from build123d import *

# Parameters (mm, degrees)
MAIN_SKETCH_W                                  = 78
MAIN_SKETCH_H                                  = 16
MAIN_SKETCH_W_2                                = 72
MAIN_SKETCH_H_2                                = 9.5
MAIN_EXTRUSION_DEPTH                           = 100
FRAISAGE_POUR_VIS_T_TE_FRAIS_E_M31_D           = 3.4
FRAISAGE_POUR_VIS_T_TE_FRAIS_E_M31_CSINK_D     = 6.3
FRAISAGE_POUR_VIS_T_TE_FRAIS_E_M31_CSINK_ANGLE = 90
R_P_TITION_LIN_AIRE1_COUNT                     = 2
R_P_TITION_LIN_AIRE1_PITCH                     = 76.6
FRAISAGE_POUR_VIS_T_TE_FRAIS_E_M32_D           = 3.4
FRAISAGE_POUR_VIS_T_TE_FRAIS_E_M32_CSINK_D     = 6.3
FRAISAGE_POUR_VIS_T_TE_FRAIS_E_M32_CSINK_ANGLE = 90
R_P_TITION_LIN_AIRE3_COUNT                     = 2
R_P_TITION_LIN_AIRE3_PITCH                     = 76.5
FRAISAGE_POUR_VIS_T_TE_FRAIS_E_M33_D           = 3.4
FRAISAGE_POUR_VIS_T_TE_FRAIS_E_M33_CSINK_D     = 6.3
FRAISAGE_POUR_VIS_T_TE_FRAIS_E_M33_CSINK_ANGLE = 90
SUPPORT_FIX_HOLE_REACH                         = 18
SUPPORT_FIX_SKETCH_R                           = 1.35


with BuildPart() as part:
    # Main-Sketch → Main-Extrusion (new body)
    with BuildSketch(Plane.XY):
        with Locations((39, 8)):
            Rectangle(MAIN_SKETCH_W, MAIN_SKETCH_H)
        with Locations((39, 8)):
            Rectangle(MAIN_SKETCH_W_2, MAIN_SKETCH_H_2, mode=Mode.SUBTRACT)
    extrude(amount=MAIN_EXTRUSION_DEPTH)

    # Fraisage pour vis à tête fraisée M31 (through all)
    with Locations(Plane.ZY):
        with Locations((9, 9.5)):
            fraisage_pour_vis_t_te_frais_e_m31 = CounterSinkHole(FRAISAGE_POUR_VIS_T_TE_FRAIS_E_M31_D / 2, FRAISAGE_POUR_VIS_T_TE_FRAIS_E_M31_CSINK_D / 2, counter_sink_angle=FRAISAGE_POUR_VIS_T_TE_FRAIS_E_M31_CSINK_ANGLE)

    # Répétition linéaire1: Fraisage pour vis à tête fraisée M31 ×2
    with Locations(*[(0, 0, i * R_P_TITION_LIN_AIRE1_PITCH) for i in range(1, R_P_TITION_LIN_AIRE1_COUNT)]):
        add(fraisage_pour_vis_t_te_frais_e_m31, mode=Mode.SUBTRACT)

    # Fraisage pour vis à tête fraisée M32 (through all)
    with Locations(Plane(origin=(78, 0, 0), x_dir=(0, 0, -1), z_dir=(1, 0, 0))):
        with Locations((-85.6, 9.5)):
            fraisage_pour_vis_t_te_frais_e_m32 = CounterSinkHole(FRAISAGE_POUR_VIS_T_TE_FRAIS_E_M32_D / 2, FRAISAGE_POUR_VIS_T_TE_FRAIS_E_M32_CSINK_D / 2, counter_sink_angle=FRAISAGE_POUR_VIS_T_TE_FRAIS_E_M32_CSINK_ANGLE)

    # Répétition linéaire3: Fraisage pour vis à tête fraisée M32 ×2
    with Locations(*[(i * R_P_TITION_LIN_AIRE3_PITCH, 0, 0) for i in range(1, R_P_TITION_LIN_AIRE3_COUNT)]):
        add(fraisage_pour_vis_t_te_frais_e_m32, mode=Mode.SUBTRACT)

    # Fraisage pour vis à tête fraisée M33 (through all)
    with Locations(Plane(origin=(78, 0, 0), x_dir=(0, 0, -1), z_dir=(1, 0, 0))):
        with Locations((-9, 9.5)):
            CounterSinkHole(FRAISAGE_POUR_VIS_T_TE_FRAIS_E_M33_D / 2, FRAISAGE_POUR_VIS_T_TE_FRAIS_E_M33_CSINK_D / 2, counter_sink_angle=FRAISAGE_POUR_VIS_T_TE_FRAIS_E_M33_CSINK_ANGLE)

    # Support-Fix-Sketch → Support-Fix-Hole (cut, up to next)
    with BuildSketch(Plane.XZ, mode=Mode.PRIVATE) as support_fix_hole_sk1:
        with Locations((68, 90)):
            Circle(SUPPORT_FIX_SKETCH_R)
    support_fix_hole_tool1 = extrude(support_fix_hole_sk1.sketch, amount=-SUPPORT_FIX_HOLE_REACH, mode=Mode.PRIVATE) & part.part
    add(support_fix_hole_tool1.solids().sort_by_distance((68, 0, 90))[0], mode=Mode.SUBTRACT)
    # Support-Fix-Sketch → Support-Fix-Hole (cut, up to next)
    with BuildSketch(Plane.XZ, mode=Mode.PRIVATE) as support_fix_hole_sk2:
        with Locations((68, 10)):
            Circle(SUPPORT_FIX_SKETCH_R)
    support_fix_hole_tool2 = extrude(support_fix_hole_sk2.sketch, amount=-SUPPORT_FIX_HOLE_REACH, mode=Mode.PRIVATE) & part.part
    add(support_fix_hole_tool2.solids().sort_by_distance((68, 0, 10))[0], mode=Mode.SUBTRACT)
    # Support-Fix-Sketch → Support-Fix-Hole (cut, up to next)
    with BuildSketch(Plane.XZ, mode=Mode.PRIVATE) as support_fix_hole_sk3:
        with Locations((10, 10)):
            Circle(SUPPORT_FIX_SKETCH_R)
    support_fix_hole_tool3 = extrude(support_fix_hole_sk3.sketch, amount=-SUPPORT_FIX_HOLE_REACH, mode=Mode.PRIVATE) & part.part
    add(support_fix_hole_tool3.solids().sort_by_distance((10, 0, 10))[0], mode=Mode.SUBTRACT)
    # Support-Fix-Sketch → Support-Fix-Hole (cut, up to next)
    with BuildSketch(Plane.XZ, mode=Mode.PRIVATE) as support_fix_hole_sk4:
        with Locations((10, 90)):
            Circle(SUPPORT_FIX_SKETCH_R)
    support_fix_hole_tool4 = extrude(support_fix_hole_sk4.sketch, amount=-SUPPORT_FIX_HOLE_REACH, mode=Mode.PRIVATE) & part.part
    add(support_fix_hole_tool4.solids().sort_by_distance((10, 0, 90))[0], mode=Mode.SUBTRACT)


solid = part.part
Could you check a few things on this model? Use its own coordinates, in mm. A direction names the side the tool comes from. Coordinates: 2 decimals unless noted, no trailing zeros. Write each loop counter-clockwise with the first axis right and the second up, starting at its lowest first coordinate (ties: lowest second). Pieces come first, ordered by that corner, then holes. Notation, with made-up numbers: (15.5, -15.75) - (26.5, -15.75) arc R18 ccw to (26.5, 1.25) - close; hole circle Ø10 at (-30.5, 46.5). An arc over 180 degrees is marked (long way). Write item = value, one per line.
1) Suppose I cut it at A-A on x = 68. Please give me the cut outline in (y, z), plus the area to 3 significant figures.
Result set:
outline = (0, 0) - (3.25, 0) - (3.25, 8.65) - (0, 8.65) - close; (0, 11.35) - (3.25, 11.35) - (3.25, 88.65) - (0, 88.65) - close; (0, 91.35) - (3.25, 91.35) - (3.25, 100) - (0, 100) - close; (12.75, 0) - (16, 0) - (16, 100) - (12.75, 100) - close
area = 632 mm2
2) Please list where these lines run through material, in increasing order: line 1 (Z direction, x = 2.3, y = 9.5); line 2 (Z direction, x = 68, y = 1.2); line 3 (X direction, y = 1.8, z = 90). Write a range as [from, to].
Result set:
line_1 = [0, 7.3], [10.7, 83.9], [87.3, 100]
line_2 = [0, 8.65], [11.35, 88.65], [91.35, 100]
line_3 = [0, 8.65], [11.35, 66.65], [69.35, 78]
3) Suppose I cut it at C-C on y = 9.5. State how many separate pieces and enclosed holes the cut face has, plus the area to 3 significant figures.
Result set:
separate_pieces = 6
enclosed_holes = 0
area = 551 mm2
4) Suppose I cut it at D-D on x = 55. Please give me the cut outline in (y, z).
Result set:
outline = (0, 0) - (3.25, 0) - (3.25, 100) - (0, 100) - close; (12.75, 0) - (16, 0) - (16, 100) - (12.75, 100) - close
5) We'd pull the mould along X, two halves only. Please class faces 1 (the flat face through (38, 3.25, 49)), 2 (the flat face through (3, 8, 49)), 3 (the flat face through (38, 16, 49)), 4 (the flat face through (0, 8, 49)): +X half, -X half, draft (parallel to the pull), parting line (faces both ways), or undercut.
Result set:
face_1 = undercut
face_2 = undercut
face_3 = draft
face_4 = -X half
6) For faces 5 (the flat face through (38, 3, 0)), 6 (the cylindrical face through (10.62, 1.6, 88.8)), which set-ups out of +Z, -Z, +X, -X, +Y, -Y let a thin tool reach every point of the face, with its end or its side?
Result set:
face_5 = -Z, +X, -X, +Y, -Y
face_6 = -Y
7) Suppose I cut it at B-B on z = 85.6. Please give me the cut outline in (x, y).
Result set:
outline = (0, 0) - (78, 0) - (78, 6.35) - (76.55, 7.8) - (75, 7.8) - (75, 3.25) - (3, 3.25) - (3, 7.8) - (1.45, 7.8) - (0, 6.35) - close; (0, 12.65) - (1.45, 11.2) - (3, 11.2) - (3, 12.75) - (75, 12.75) - (75, 11.2) - (76.55, 11.2) - (78, 12.65) - (78, 16) - (0, 16) - close
8) Will these pins go through, and if not, where does the flat tip stop? pin 1 Ø2.5 at (x, z) = (68, 90) entering from -Y; pin 2 Ø4 at (y, z) = (9.5, 9) entering from -X; pin 3 Ø5.5 at (y, z) = (9.5, 85.6) entering from -X.
Result set:
pin_1 = 12.75
pin_2 = 1.15
pin_3 = 0.4
